The model under review builds one solid part; all positions refer to its coordinate system, in mm. Face numbers are marked on the shaded views. Coordinates: 2 decimals unless noted, no trailing zeros. Loops run counter-clockwise (first coordinate to the right, second up) from the corner with the lowest first, then second, coordinate; pieces in that order, holes last. Notation, with made-up numbers: M 89,-34 L 143,-34 A24 ccw 143,2 Z; hole C -10,-35 d7. An arc over 180 degrees is marked long. Use CSV: the item, a comma, the result in double quotes. Start each with the question number.
from build123d import *

# Parameters (mm, degrees)
SKETCH1_W           = 100
SKETCH1_H           = 40
BOSS_EXTRUDE2_DEPTH = 20
SKETCH3_R           = 12.5
CUT_EXTRUDE1_DEPTH  = 100
SKETCH4_R           = 2
SKETCH4_R_2         = 1.5
CUT_EXTRUDE2_DEPTH  = 20
SKETCH5_R           = 10
CUT_EXTRUDE3_DEPTH  = 20


with BuildPart() as part:
    # Sketch1 → Boss-Extrude2 (new body)
    with BuildSketch(Plane.XY):
        Rectangle(SKETCH1_W, SKETCH1_H)
    extrude(amount=BOSS_EXTRUDE2_DEPTH)

    # Sketch3 → Cut-Extrude1 (cut)
    with BuildSketch(Plane(origin=(50, 0, 0), x_dir=(0, 0, -1), z_dir=(1, 0, 0))):
        with Locations((-20, 0)):
            Circle(SKETCH3_R)
    extrude(amount=-CUT_EXTRUDE1_DEPTH, mode=Mode.SUBTRACT)

    # Sketch4 → Cut-Extrude2 (cut)
    with BuildSketch(Plane.XY.offset(20)):
        with Locations((-20, 16.25)):
            Circle(SKETCH4_R)
        with Locations((-30, 16.25)):
            Circle(SKETCH4_R_2)
        with Locations((-40, 16.25)):
            Circle(SKETCH4_R)
        with Locations((30, 16.25)):
            Circle(SKETCH4_R_2)
        with Locations((40, 16.25)):
            Circle(SKETCH4_R)
        with Locations((20, 16.25)):
            Circle(SKETCH4_R)
        with Locations((-40, -16.25)):
            Circle(SKETCH4_R)
        with Locations((-30, -16.25)):
            Circle(SKETCH4_R_2)
        with Locations((-20, -16.25)):
            Circle(SKETCH4_R)
        with Locations((20, -16.25)):
            Circle(SKETCH4_R)
        with Locations((30, -16.25)):
            Circle(SKETCH4_R_2)
        with Locations((40, -16.25)):
            Circle(SKETCH4_R)
    extrude(amount=-CUT_EXTRUDE2_DEPTH, mode=Mode.SUBTRACT)

    # Sketch5 → Cut-Extrude3 (cut)
    with BuildSketch(Plane(origin=(0, 0, 0), x_dir=(-1, 0, 0), z_dir=(0, 0, -1))):
        Circle(SKETCH5_R)
    extrude(amount=-CUT_EXTRUDE3_DEPTH, mode=Mode.SUBTRACT)


solid = part.part
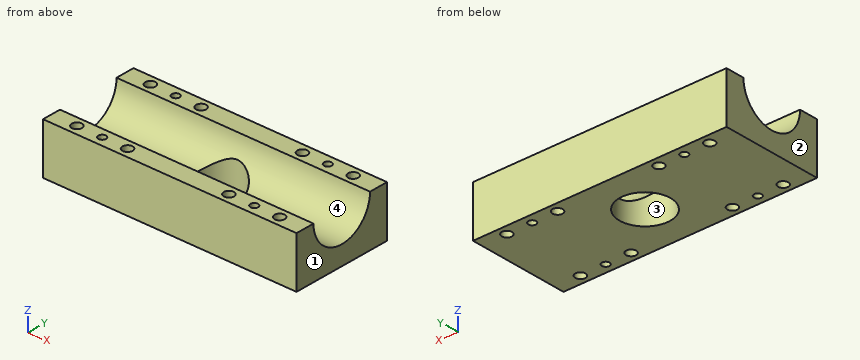
1. Add section B-B (x = 30). Write out the cut boundary in (y, z).
2. To check wall thickness, follow line 1 along X through (y, z) = (-14.5, 11.5); line 2 along Y through (x, z) = (-40, 12.75); line 3 along X through (y, z) = (0.5, 3.5). State the ranges of each line that lie inside material, in increasing order.
3. Add section D-D (y = -16.25). Write out the cut boundary in (x, z), plus the area to 3 significant figures.
4. Draft analysis for pull direction X (two halves, no side actions). For the marked faces 1, 2, 3 and 4, state which applies: released by +X, released by -X, zero draft, split by the parting line, or undercut.
5. Add section A-A (z = 18.25). Give the number of separate pieces and of enclosed holes in the cut face, plus the area to 3 significant figures.
6. Insertion check: pin 1 Ø3.5 at (x, y) = (30, 16.25) entering from +Z. The pin has a flat end and moves straight along its axis. Give the tip position at first contact, or say it passes through.
Solved:
1,outline,"M -20,0 L -17.75,0 L -17.75,20 L -20,20 Z; M -14.75,0 L 14.75,0 L 14.75,20 L 12.5,20 A12.5 cw -12.5,20 L -14.75,20 Z; M 17.75,0 L 20,0 L 20,20 L 17.75,20 Z"
2,line 1,"x = -50 to -40.97, -39.03 to -20.97, -19.03 to 19.03, 20.97 to 39.03, 40.97 to 50"
2,line 2,"y = -20 to -18.25, -14.25 to -10.18, 10.18 to 14.25, 18.25 to 20"
2,line 3,"x = -50 to -9.99, 9.99 to 50"
3,outline,"M -50,0 L -42,0 L -42,20 L -50,20 Z; M -38,0 L -31.5,0 L -31.5,20 L -38,20 Z; M -28.5,0 L -22,0 L -22,20 L -28.5,20 Z; M -18,0 L 18,0 L 18,20 L -18,20 Z; M 22,0 L 28.5,0 L 28.5,20 L 22,20 Z; M 31.5,0 L 38,0 L 38,20 L 31.5,20 Z; M 42,0 L 50,0 L 50,20 L 42,20 Z"
3,area,"1,560 mm^2"
4,face 1,"released by +X"
4,face 2,"released by -X"
4,face 3,"undercut"
4,face 4,"zero draft"
5,separate pieces,"2"
5,enclosed holes,"12"
5,area,"1,400 mm^2"
6,pin 1,"stops at z = 20"
